Part print with two shaded views. Sizes in mm from the minimum x, y, z corner. Round coordinates to 2 decimals unless told otherwise and drop trailing zeros. Write each loop counter-clockwise with the first axis right and the second up, starting at its lowest first coordinate (ties: lowest second). Pieces come first, ordered by that corner, then holes. Notation, with made-up numbers: (26.25, 66) -> (59.25, 66) arc R15 ccw to (59.25, 76) -> close; hole circle Ø7 at (-29.5, 4.5). An arc over 180 degrees is marked (long way). Answer in a Markdown table with one row per item.
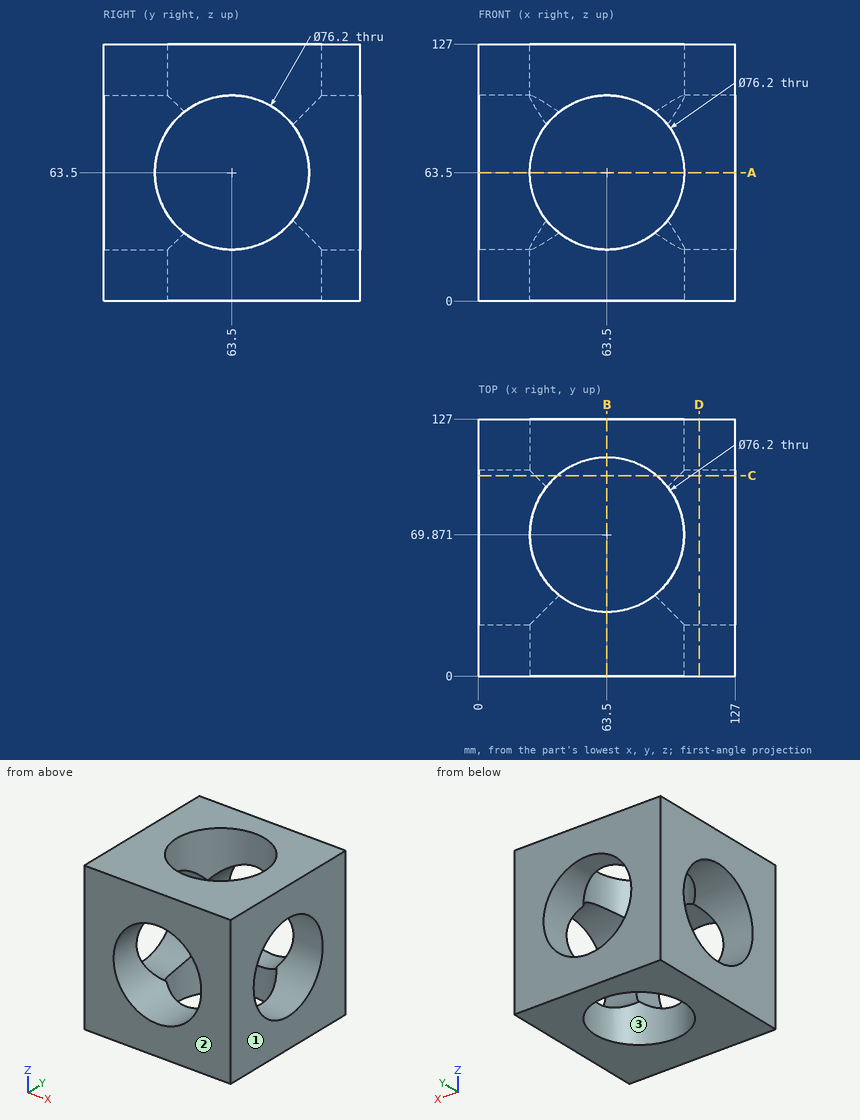
Q1. Saw through at C-C on y = 99. Write the cut outline in (x, z), plus the area to 3 significant figures.
A:
| item | result |
|---|---|
| outline | (0, 0) -> (38.94, 0) -> (38.94, 34.37) arc R38.1 cw to (28, 49.67) -> (0, 49.67) -> close; (0, 77.33) -> (28, 77.33) arc R38.1 cw to (38.94, 92.63) -> (38.94, 127) -> (0, 127) -> close; (88.06, 0) -> (127, 0) -> (127, 49.67) -> (99, 49.67) arc R38.1 cw to (88.06, 34.37) -> close; (88.06, 92.63) arc R38.1 cw to (99, 77.33) -> (127, 77.33) -> (127, 127) -> (88.06, 127) -> close |
| area | 7,340 mm² |
Q2. Saw through at D-D on x = 109. Write the cut outline in (y, z), plus the area to 3 significant figures.
A:
| item | result |
|---|---|
| outline | (0, 0) -> (127, 0) -> (127, 127) -> (0, 127) -> close; hole circle Ø76.2 at (63.5, 63.5) |
| area | 11,600 mm² |
Q3. Saw through at B-B on x = 63.5. Write the cut outline in (y, z).
A:
| item | result |
|---|---|
| outline | (0, 0) -> (31.77, 0) -> (31.77, 25.4) -> (0, 25.4) -> close; (0, 101.6) -> (31.77, 101.6) -> (31.77, 127) -> (0, 127) -> close; (107.97, 0) -> (127, 0) -> (127, 25.4) -> (107.97, 25.4) -> close; (107.97, 101.6) -> (127, 101.6) -> (127, 127) -> (107.97, 127) -> close |
Q4. Saw through at A-A on z = 63.5. Write the cut outline in (x, y).
A:
| item | result |
|---|---|
| outline | (0, 0) -> (25.4, 0) -> (25.4, 25.4) -> (0, 25.4) -> close; (0, 101.6) -> (25.4, 101.6) -> (25.4, 127) -> (0, 127) -> close; (101.6, 0) -> (127, 0) -> (127, 25.4) -> (101.6, 25.4) -> close; (101.6, 101.6) -> (127, 101.6) -> (127, 127) -> (101.6, 127) -> close |
Q5. Wall check: line 1 (Y direction, x = 115, z = 63); line 2 (Y direction, x = 63.5, z = 111.5). Give the ranges that are in metal, low to high. Write a range as [from, to].
A:
| item | result |
|---|---|
| line 1 | [0, 25.4], [101.6, 127] |
| line 2 | [0, 31.77], [107.97, 127] |
Q6. Two-plate mould, pull along Y, no slides. Class the marked faces 1, 2 and 3: released by +Y, released by -Y, zero draft, split by the parting line, or undercut.
A:
| item | result |
|---|---|
| face 1 | zero draft |
| face 2 | released by -Y |
| face 3 | undercut |
